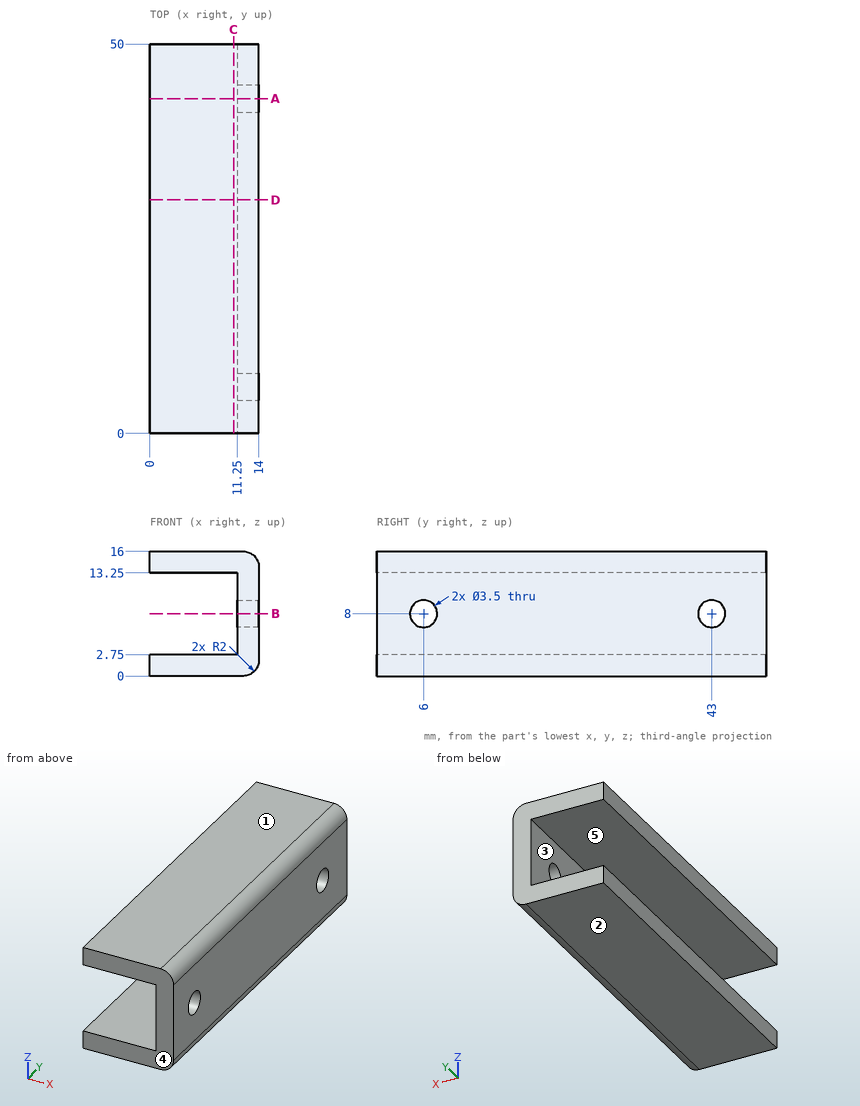
Answer from the drawing. Dimensions are ordinates in mm from the lowest x, y and z of the part. A direction names the side the tool comes from. Round coordinates to 2 decimals unless told otherwise and drop trailing zeros. Loops run counter-clockwise (first coordinate to the right, second up) from the corner with the lowest first, then second, coordinate; pieces in that order, holes last.
Q1. Which of the six approach directions +Z, -Z, +X, -X, +Y, -Y give full straight-line access (tool end or side, diameter ignored) to the marked faces 4 and 5?
Q2. Section D-D on y = 30 is taken. Write down the section's boundary in (x, z).
Q3. Determine the mould class of the marked faces 1, 2 and 3 for opening direction Z: released by +Z, released by -Z, zero draft, split by the parting line, or undercut.
Q4. Each of these flat-tipped pins is pushed along its axis until it touches: pin 1 (4 mm diameter, centred on y = 30, z = 10.5, fed in from -X); pin 2 (1 mm diameter, centred on x = 6, z = 11, fed in from -Y). Where does it stop, or does it pass through?
Q5. Consider probe 1 along Y at (x, z) = (13.25, 8); probe 2 along Z at (x, y) = (1.5, 20); probe 3 along X at (y, z) = (10, 12.5). Determine where each line is inside the solid, lowest interval first.
Q6. Section A-A on y = 43 is taken. Write down the section's boundary in (x, z).
Q7. Section B-B on z = 8 is taken. Write down the section's boundary in (x, y), and give its area (3 significant figures).
Q8. Section C-C on x = 10.75 is taken. Write down the section's boundary in (y, z).
Output:
1. face 4: +Z, -Z, +X, -X, -Y
1. face 5: -X, +Y, -Y
2. outline: (0, 0) - (12, 0) arc R2 ccw to (14, 2) - (14, 14) arc R2 ccw to (12, 16) - (0, 16) - (0, 13.25) - (11.25, 13.25) - (11.25, 2.75) - (0, 2.75) - close
3. face 1: released by +Z
3. face 2: released by -Z
3. face 3: undercut
4. pin 1: stops at x = 11.25
4. pin 2: passes through
5. probe 1: y = 0 to 4.25, 7.75 to 41.25, 44.75 to 50
5. probe 2: z = 0 to 2.75, 13.25 to 16
5. probe 3: x = 11.25 to 14
6. outline: (0, 0) - (12, 0) arc R2 ccw to (14, 2) - (14, 6.25) - (11.25, 6.25) - (11.25, 2.75) - (0, 2.75) - close; (0, 13.25) - (11.25, 13.25) - (11.25, 9.75) - (14, 9.75) - (14, 14) arc R2 ccw to (12, 16) - (0, 16) - close
7. outline: (11.25, 0) - (14, 0) - (14, 4.25) - (11.25, 4.25) - close; (11.25, 7.75) - (14, 7.75) - (14, 41.25) - (11.25, 41.25) - close; (11.25, 44.75) - (14, 44.75) - (14, 50) - (11.25, 50) - close
7. area: 118 mm2
8. outline: (0, 0) - (50, 0) - (50, 2.75) - (0, 2.75) - close; (0, 13.25) - (50, 13.25) - (50, 16) - (0, 16) - close
